Can you work these out from the model? Positions are in its coordinate system, mm. A direction names the side the tool comes from. Coordinates: 2 decimals unless noted, no trailing zeros. Loops run counter-clockwise (first coordinate to the right, second up) from the corner with the lowest first, then second, coordinate; pieces in that order, holes last.
```python
from build123d import *

# Parameters (mm, degrees)
BOSS_EXTRUDE1_DEPTH  = 4.5
BOSS_EXTRUDE2_DEPTH  = 4
CHAMFER2_2_DEPTH     = 4.2
CHAMFER2_START       = 4.2
CHAMFER2_3_OUTLINE_R = 8.8
CHAMFER2_3_DEPTH     = 3.8
SKETCH4_R            = 3
CUT_EXTRUDE1_DEPTH   = 103.673405573
CUT_EXTRUDE2_DEPTH   = 4.9
CUT_EXTRUDE3_DEPTH   = 5


with BuildPart() as part:
    # Sketch2 → Boss-Extrude1 (new body)
    with BuildSketch(Plane.XY):
        with BuildLine():
            Line((0, 12.6), (88.98281443, 12.6))
            ThreePointArc((88.98281443, 12.6), (101.58281443, 0), (88.98281443, -12.6))
            Line((88.98281443, -12.6), (0, -12.6))
            ThreePointArc((0, -12.6), (-12.6, 0), (0, 12.6))
        make_face()
    extrude(amount=BOSS_EXTRUDE1_DEPTH)

    # Sketch3 → Boss-Extrude2 (add)
    with BuildSketch(Plane.XY.offset(8)):
        with BuildLine():
            Line((-0.708592785, -8.85), (89.691407215, -8.85))
            ThreePointArc((89.691407215, -8.85), (98.541407215, 0), (89.691407215, 8.85))
            Line((89.691407215, 8.85), (-0.708592785, 8.85))
            ThreePointArc((-0.708592785, 8.85), (-9.558592785, 0), (-0.708592785, -8.85))
        make_face()
    extrude(amount=-BOSS_EXTRUDE2_DEPTH)

    # Chamfer2: read off the stored shape, not the designer's step
    # Chamfer2 outline → Chamfer2 (revolve)
    with BuildSketch(Plane(origin=(88.98281443, 0, 0), x_dir=(1, 0, 0), z_dir=(0, -1, 0))):
        Polygon((12.6, 4.2), (8.8, 8), (8.8, 4.2), align=None)
    revolve(axis=Axis((88.98281443, 0, 0), (0, 0, 1)))

    # Chamfer2 2 outline → Chamfer2 2 (add)
    with BuildSketch(Plane.XY):
        with BuildLine():
            ThreePointArc((0, 12.6), (-12.6, 0), (0, -12.6))
            Line((0, -12.6), (88.98281443, -12.6))
            ThreePointArc((88.98281443, -12.6), (101.58281443, 0), (88.98281443, 12.6))
            Line((88.98281443, 12.6), (0, 12.6))
        make_face()
    extrude(amount=CHAMFER2_2_DEPTH)

    # Chamfer2 3 outline → Chamfer2 3 (add)
    with BuildSketch(Plane.XY.offset(CHAMFER2_START)):
        with Locations((88.98281443, 0)):
            Circle(CHAMFER2_3_OUTLINE_R)
    extrude(amount=CHAMFER2_3_DEPTH)

    # Chamfer2 4: loft between two sections, ruled curve by curve
    chamfer2_4_from = [
        Edge.make_three_point_arc((0, -8.8, 8), (-6.222539674, -6.222539674, 8), (-8.8, 0, 8)),
        Edge.make_three_point_arc((-8.8, 0, 8), (-6.222539674, 6.222539674, 8), (0, 8.8, 8)),
        Edge.make_line((88.98281443, 8.8, 8), (0, 8.8, 8)),
        Edge.make_line((0, -8.8, 8), (88.98281443, -8.8, 8)),
        Edge.make_line((88.98281443, -8.8, 8), (88.98281443, 8.8, 8)),
    ]
    chamfer2_4_to = [
        Edge.make_three_point_arc((0, -12.6, 4.2), (-8.909545443, -8.909545443, 4.2), (-12.6, 0, 4.2)),
        Edge.make_three_point_arc((-12.6, 0, 4.2), (-8.909545443, 8.909545443, 4.2), (0, 12.6, 4.2)),
        Edge.make_line((88.98281443, 12.6, 4.2), (0, 12.6, 4.2)),
        Edge.make_line((0, -12.6, 4.2), (88.98281443, -12.6, 4.2)),
        Edge.make_line((88.98281443, -12.6, 4.2), (88.98281443, 12.6, 4.2)),
    ]
    chamfer2_4 = Solid(Shell([*[Face.make_surface_from_curves(chamfer2_4_from[k], chamfer2_4_to[k]) for k in range(5)], Face(Wire(chamfer2_4_from)), Face(Wire(chamfer2_4_to))]))
    add(chamfer2_4)

    # Sketch4 → Cut-Extrude1 (cut, through all)
    with BuildSketch(Plane.XY):
        with Locations((88.98281443, 0)):
            Circle(SKETCH4_R)
        Circle(SKETCH4_R)
    extrude(amount=CUT_EXTRUDE1_DEPTH, mode=Mode.SUBTRACT)

    # Sketch5 → Cut-Extrude2 (cut)
    with BuildSketch(Plane.XY.offset(8)):
        Polygon((3, -5), (-3, -5), (-5.8, 0), (-3, 5), (3, 5), (5.8, 0), align=None)
        Polygon((83.18281443, 0), (85.98281443, 5), (91.98281443, 5), (94.78281443, 0), (91.98281443, -5), (85.98281443, -5), align=None)
    extrude(amount=-CUT_EXTRUDE2_DEPTH, mode=Mode.SUBTRACT)

    # Sketch6 → Cut-Extrude3 (cut)
    with BuildSketch(Plane.XY):
        with BuildLine():
            Line((70.338627057, 7.052928589), (72.459947401, 4.931608246))
            Line((72.459947401, 4.931608246), (67.492805249, -0.035533906))
            ThreePointArc((67.492805249, -0.035533906), (65.870688505, -1.119397663), (63.957271343, -1.5))
            Line((63.957271343, -1.5), (55.182814215, -1.5))
            Line((55.182814215, -1.5), (55.182814215, -3.5))
            Line((55.182814215, -3.5), (52.382814215, -3.5))
            Line((52.382814215, -3.5), (52.382814215, -1.5))
            Line((52.382814215, -1.5), (45.961101061, -1.5))
            ThreePointArc((45.961101061, -1.5), (44.491407215, -2.1), (43.021713369, -1.5))
            Line((43.021713369, -1.5), (26.268183774, -1.5))
            ThreePointArc((26.268183774, -1.5), (24.354766612, -1.880602337), (22.732649868, -2.964466094))
            Line((22.732649868, -2.964466094), (18.644187373, -7.052928589))
            Line((18.644187373, -7.052928589), (16.522867029, -4.931608246))
            Line((16.522867029, -4.931608246), (21.490009181, 0.035533906))
            ThreePointArc((21.490009181, 0.035533906), (23.112125925, 1.119397663), (25.025543087, 1.5))
            Line((25.025543087, 1.5), (43.021713369, 1.5))
            ThreePointArc((43.021713369, 1.5), (44.491407215, 2.1), (45.961101061, 1.5))
            Line((45.961101061, 1.5), (62.714630656, 1.5))
            ThreePointArc((62.714630656, 1.5), (64.628047818, 1.880602337), (66.250164562, 2.964466094))
            Line((66.250164562, 2.964466094), (70.338627057, 7.052928589))
        make_face()
    extrude(amount=CUT_EXTRUDE3_DEPTH, mode=Mode.SUBTRACT)


solid = part.part
```
Item 1: We'd pull the mould along Y, two halves only. Please class faces 4 (the face through (44, -12.6, 2)), 5 (the face through (45, 12.6, 2)), 6 (the face through (71.38, 6.01, 2.46)), 7 (the face through (44.5, -2.1, 2.5)): +Y half, -Y half, draft (parallel to the pull), parting line (faces both ways), or undercut.
Results are:
face 4: -Y half
face 5: +Y half
face 6: undercut
face 7: undercut
Item 2: I'm going to push flat-ended pins straight in: P1, Ø8, axis at x = 88.98, y = 0, coming from the +Z side; P2, Ø1, axis at y = -2.5, z = 3.5, coming from the -X side; P3, Ø2, axis at y = -9.5, z = 5, coming from the +X side. Where does each tip first touch, or does it pass through?
Results are:
P1: stops at z = 3.1
P2: stops at x = -12.44
P3: stops at x = 97.9
Item 3: I need wall thicknesses on line 1 along Y through (x, z) = (47, 1); line 2 along X through (y, z) = (0, 2); line 3 along X through (y, z) = (-0.25, 2.25). Which ranges of each line are inside material? Lowest first, please.
Results are:
line 1: y = -12.6 to -1.5, 1.5 to 12.6
line 2: x = -12.6 to -3, 3 to 21.45, 67.53 to 85.98, 91.98 to 101.58
line 3: x = -12.6 to -2.99, 2.99 to 21.2, 67.26 to 85.99, 91.97 to 101.58
Item 4: Suppose I cut it at A-A, the plane z = 1.75. Please give me the cut outline in (x, y).
Results are:
outline: (0, -12.6) - (88.98, -12.6) arc R12.6 ccw to (88.98, 12.6) - (0, 12.6) arc R12.6 ccw to start; hole circle Ø6 at (0, 0); hole (16.52, -4.93) - (18.64, -7.05) - (22.73, -2.96) arc R5 cw to (26.27, -1.5) - (43.02, -1.5) arc R2.1 ccw to (45.96, -1.5) - (52.38, -1.5) - (52.38, -3.5) - (55.18, -3.5) - (55.18, -1.5) - (63.96, -1.5) arc R5 ccw to (67.49, -0.04) - (72.46, 4.93) - (70.34, 7.05) - (66.25, 2.96) arc R5 cw to (62.71, 1.5) - (45.96, 1.5) arc R2.1 ccw to (43.02, 1.5) - (25.03, 1.5) arc R5 ccw to (21.49, 0.04) - close; hole circle Ø6 at (88.98, 0)
Item 5: On a 3-axis mill with a long thin cutter (end or side, diameter ignored), from which of +Z, -Z, +X, -X, +Y, -Y can I reach the whole of each face in a straight line? I mean faces 1 (the face through (93.4, -2.47, 5.58)), 2 (the face through (-12.597, 0.277, 2.071)), 3 (the face through (34, 1.5, 2)). Say none if no direction works.
Results are:
face 1: +Z
face 2: +Z, -Z, -X
face 3: -Z
